Autodesk Inventor part; units mm, degrees
ref_plane "YZ Plane" through (0, 0, 0) normal (1, 0, 0) x (0, 1, 0)
ref_plane "XZ Plane" through (0, 0, 0) normal (0, 1, 0) x (-1, 0, 0)
ref_plane "XY Plane" through (0, 0, 0) normal (0, 0, 1) x (1, 0, 0)
sketch "Sketch1" plane through (0, 0, 0) normal (0, 0, 1) x (1, 0, 0)
  line L0 (-3.5, -5) -> (3.5, -5)
  line L1 (3.5, -5) -> (3.5, 5)
  line L2 (3.5, 5) -> (-3.5, 5)
  line L3 (-3.5, 5) -> (-3.5, -5)
  line L4 (-3.5, -5) -> (3.5, 5) construction
  line L5 (3.5, -5) -> (-3.5, 5) construction
  point P0 (0, 0)
  dimension "d0" = 7
  dimension "d1" = 10
extrude "Extrusion1" add sketch "Sketch1" along normal blind 250
sketch "Sketch2" plane through (-3.5, -5, 0) normal (-1, 0, 0) x (0, 0, 1)
  line L0 (0, 0) -> (250, 0)
  line L1 (0, 10) -> (250, 10)
  line L2 (65, 0) -> (70, 0)
  line L3 (70, 0) -> (70, 10)
  line L4 (70, 10) -> (65, 10)
  line L5 (65, 10) -> (65, 0)
  point P0 (0, 5)
  dimension "d4" = 5
  dimension "d5" = 65
extrude "Extrusion2" add sketch "Sketch2" along normal blind 100
fillet "Fillet1" radius 2 2 edges at (-103.5, 0, 65) (-103.5, 0, 70)
sketch "Sketch3" plane through (3.5, 5, 250) normal (0, 1, 0) x (1, 0, 0)
  circle A0 centre (-103.2335, 182.6391) radius 2
  point P0 (-3.5, 250)
  dimension "d9" = 4
extrude "Extrusion3" cut sketch "Sketch3" against normal through all
properties part number "support_rod_right"
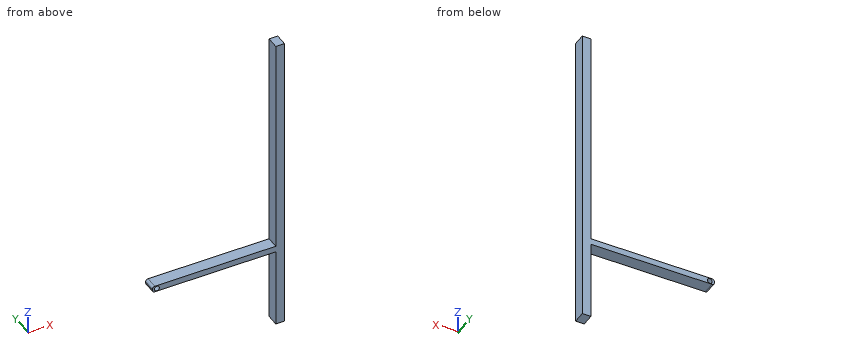
The listing builds one solid part. Answer for the finished solid, in the listing's coordinates (mm). Round coordinates to 2 decimals unless told otherwise and drop trailing zeros. Write each loop counter-clockwise with the first axis right and the second up, starting at its lowest first coordinate (ties: lowest second). Pieces come first, ordered by that corner, then holes. Notation, with made-up numbers: M 85,72.25 L 122,72.25 A28 cw 122,106.25 Z; hole C 31.5,61.25 d3. An arc over 180 degrees is marked long. Write each question's results on one line, items separated by ' | '. Start each with the question number.
(1) The part is cut by section A-A, the plane y = 2.5. Write down the section's boundary in (x, z).
(2) Each of these flat-tipped pins is pushed along its axis until it touches: P1, Ø5, axis at y = -2.5, z = 28.5, coming from the -X side; P2, Ø6, axis at x = -40.5, y = 2, coming from the +Z side; P3, Ø2, axis at x = -47, y = 0.5, coming from the -Z side. Where does it stop, or does it pass through?
(3) The part is cut by section C-C, the plane z = 163. Write down the section's boundary in (x, y), and give its area (3 significant figures).
(4) The part is cut by section B-B, the plane x = -25.5. Write down the section's boundary in (y, z).
(5) Find the intervals of material crossed by line 1 (Z direction, x = -14.5, y = 0.5); line 2 (X direction, y = -2.75, z = 172), in increasing order.
Worked answers:
1) outline: M -103.5,67 A2 ccw -101.5,65 L -3.5,65 L -3.5,0 L 3.5,0 L 3.5,250 L -3.5,250 L -3.5,70 L -101.5,70 A2 ccw -103.5,68 Z; hole C -99.73,67.36 d4
2) P1: stops at x = -3.5 | P2: stops at z = 70 | P3: stops at z = 65
3) outline: M -3.5,-5 L 3.5,-5 L 3.5,5 L -3.5,5 Z | area: 70.0 mm²
4) outline: M -5,65 L 5,65 L 5,70 L -5,70 Z
5) line 1: z = 65 to 70 | line 2: x = -3.5 to 3.5
